The listing builds one solid part. Answer for the finished solid, in the listing's coordinates (mm). A direction names the side the tool comes from. Coordinates: 2 decimals unless noted, no trailing zeros. Order: outer loops, then holes, each group sorted by start corner. A loop starts at its lowest first (then second) coordinate and runs counter-clockwise, first axis right, second up. Notation, with made-up numbers: (-34, 20.5) -> (-9, 20.5) arc R26 cw to (-9, 41.5) -> close; hole circle Ø5 at (37, 52.5). An arc over 180 degrees is marked (long way). Return JSON: item names as keys, results as strings.
```python
from build123d import *

# Parameters (mm, degrees)
CYLINDER008_R           = 6
CYLINDER008_DEPTH       = 1.5
PRISM001_DEPTH          = 5
FUSION006003_ROLL_ANGLE = -90
CYLINDER006_R           = 3
CYLINDER006_DEPTH       = 25
CYLINDER007_R           = 5
CYLINDER007_DEPTH       = 4
FUSION006002_ROLL_ANGLE = 90
CYLINDER005_R           = 9.5
CYLINDER005_DEPTH       = 6
CYLINDER005_ROLL_ANGLE  = 90
CYLINDER009_R           = 6
CYLINDER009_DEPTH       = 1.5
CYLINDER009_ROLL_ANGLE  = 90


with BuildPart() as cylinder006:
    # Cylinder008 → Cylinder008 (new body)
    with BuildSketch(Plane.XY):
        Circle(CYLINDER008_R)
    extrude(amount=CYLINDER008_DEPTH)


with BuildPart() as fusion006003:
    # Prism001 → Prism001 (new body)
    with BuildSketch(Plane.XY.offset(1.5)):
        Polygon((5.5, 0), (2.75, 4.76314), (-2.75, 4.76314), (-5.5, 0), (-2.75, -4.76314), (2.75, -4.76314), align=None)
    extrude(amount=PRISM001_DEPTH)

    # Fusion006003: union Cylinder006
    add(cylinder006.part)


with BuildPart() as fusion006003_1:
    # Fusion006003 roll: moved
    add(fusion006003.part.rotate(Axis((0, 0, 0), (1, 0, 0)), FUSION006003_ROLL_ANGLE))


with BuildPart() as fusion006003_2:
    # Fusion006003 placement: moved
    add(fusion006003_1.part.moved(Location((0, 10, 14))))


with BuildPart() as cylinder004:
    # Cylinder006 → Cylinder006 (new body)
    with BuildSketch(Plane.XY):
        Circle(CYLINDER006_R)
    extrude(amount=CYLINDER006_DEPTH)


with BuildPart() as belt_bearing_screw:
    # Cylinder007 → Cylinder007 (new body)
    with BuildSketch(Plane.XY.offset(25)):
        Circle(CYLINDER007_R)
    extrude(amount=CYLINDER007_DEPTH)

    # Fusion006002: union Cylinder004
    add(cylinder004.part)


with BuildPart() as belt_bearing_screw_1:
    # Fusion006002 roll: moved
    add(belt_bearing_screw.part.rotate(Axis((0, 0, 0), (1, 0, 0)), FUSION006002_ROLL_ANGLE))


with BuildPart() as belt_bearing_screw_2:
    # Fusion006002 placement: moved
    add(belt_bearing_screw_1.part.moved(Location((0, 22.5, 14))))


with BuildPart() as belt_bearing:
    # Cylinder005 → Cylinder005 (new body)
    with BuildSketch(Plane.XY):
        Circle(CYLINDER005_R)
    extrude(amount=CYLINDER005_DEPTH)


with BuildPart() as belt_bearing_1:
    # Cylinder005 roll: moved
    add(belt_bearing.part.rotate(Axis((0, 0, 0), (1, 0, 0)), CYLINDER005_ROLL_ANGLE))


with BuildPart() as belt_bearing_2:
    # Cylinder005 placement: moved
    add(belt_bearing_1.part.moved(Location((0, 3.5, 14))))


with BuildPart() as belt_holder:
    # Cylinder009 → Cylinder009 (new body)
    with BuildSketch(Plane.XY):
        Circle(CYLINDER009_R)
    extrude(amount=CYLINDER009_DEPTH)


with BuildPart() as belt_holder_1:
    # Cylinder009 roll: moved
    add(belt_holder.part.rotate(Axis((0, 0, 0), (1, 0, 0)), CYLINDER009_ROLL_ANGLE))


with BuildPart() as belt_holder_2:
    # Cylinder009 placement: moved
    add(belt_holder_1.part.moved(Location((0, 5, 14))))

    # Fusion006004: union Fusion006003, Belt_Bearing_Screw, Belt_Bearing
    add(fusion006003_2.part)
    add(belt_bearing_screw_2.part)
    add(belt_bearing_2.part)


solid = belt_holder_2.part
```
Item 1: Flat-ended cylindrical pins translate along their axes: pin 1 (4 mm diameter, centred on x = 0, y = 13, fed in from +Z); pin 2 (2 mm diameter, centred on x = 3, y = 9.5, fed in from +Z); pin 3 (1.5 mm diameter, centred on x = 0, y = 14.5, fed in from -Z). Find the tip coordinate at first contact, or state that the pin passes through.
Answer list:
{"pin 1": "z = 20", "pin 2": "z = 19.61", "pin 3": "z = 9.24"}
Item 2: The part is cut by section B-B on z = 8.5. Determine the outline of the cut face in (x, y).
Answer list:
{"outline": "(-7.75, -2.5) -> (7.75, -2.5) -> (7.75, 3.5) -> (2.4, 3.5) -> (2.4, 5) -> (-2.4, 5) -> (-2.4, 3.5) -> (-7.75, 3.5) -> close; (-2.4, 10) -> (2.4, 10) -> (2.4, 11.5) -> (-2.4, 11.5) -> close"}
Item 3: Find the intervals of material crossed by probe 1 along Y at (x, z) = (-1.25, 10.5); probe 2 along Z at (x, y) = (-0.5, 14); probe 3 along Y at (x, z) = (4.5, 20.5), in increasing order.
Answer list:
{"probe 1": "-6.5 to 5, 10 to 16.5", "probe 2": "9.24 to 18.76", "probe 3": "-2.5 to 3.5"}
Item 4: Which of the six approach directions +Z, -Z, +X, -X, +Y, -Y give full straight-line access (tool end or side, diameter ignored) to faces 4 (the flat face through (4.11, 13.96, 16.41)), 5 (the flat face through (-4.144, 13.965, 16.348)), 6 (the flat face through (-0.1, 3.5, 7.8))?
Answer list:
{"face 4": "+Z, +X, +Y", "face 5": "+Z, -X, +Y", "face 6": "+Y"}
Item 5: The part is cut by section A-A on x = 3.5. Determine the outline of the cut face in (y, z), plus the area to 3 significant figures.
Answer list:
{"outline": "(-6.5, 10.43) -> (-2.5, 10.43) -> (-2.5, 5.17) -> (3.5, 5.17) -> (3.5, 9.13) -> (5, 9.13) -> (5, 18.87) -> (3.5, 18.87) -> (3.5, 22.83) -> (-2.5, 22.83) -> (-2.5, 17.57) -> (-6.5, 17.57) -> close; (10, 9.13) -> (11.5, 9.13) -> (11.5, 10.54) -> (16.5, 10.54) -> (16.5, 17.46) -> (11.5, 17.46) -> (11.5, 18.87) -> (10, 18.87) -> close", "area": "198 mm2"}
Item 6: The part is cut by section C-C on x = 0. Determine the outline of the cut face in (y, z), plus the area to 3 significant figures.
Answer list:
{"outline": "(-6.5, 9) -> (-2.5, 9) -> (-2.5, 4.5) -> (3.5, 4.5) -> (3.5, 8) -> (5, 8) -> (5, 11) -> (10, 11) -> (10, 8) -> (11.5, 8) -> (11.5, 9.24) -> (16.5, 9.24) -> (16.5, 11) -> (22.5, 11) -> (22.5, 17) -> (16.5, 17) -> (16.5, 18.76) -> (11.5, 18.76) -> (11.5, 20) -> (10, 20) -> (10, 17) -> (5, 17) -> (5, 20) -> (3.5, 20) -> (3.5, 23.5) -> (-2.5, 23.5) -> (-2.5, 19) -> (-6.5, 19) -> close", "area": "304 mm2"}
Item 7: The part is cut by section D-D on y = 1.5. Determine the outline of the cut face in (x, z).
Answer list:
{"outline": "circle Ø19 at (0, 14)"}
Item 8: Determine the mould class of faces 1 (the cylindrical face through (-1.08, -4.47, 9.12)), 2 (the flat face through (2.4, 16.5, 16.1)), 3 (the cylindrical face through (-0.65, 7.54, 11.07)) for opening direction Y: pulls with the +Y half, pulls with the -Y half, needs draft (parallel to the pull), parting line crosses it, or undercut.
Answer list:
{"face 1": "needs draft", "face 2": "pulls with the +Y half", "face 3": "undercut"}
